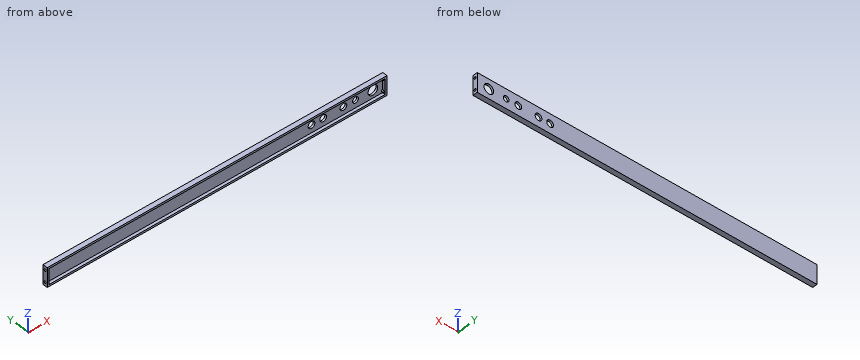
Autodesk Inventor part; units mm, degrees
ref_plane "YZ Plane" through (0, 0, 0) normal (1, 0, 0) x (0, 1, 0)
ref_plane "XZ Plane" through (0, 0, 0) normal (0, 1, 0) x (-1, 0, 0)
ref_plane "XY Plane" through (0, 0, 0) normal (0, 0, 1) x (1, 0, 0)
sketch "スケッチ1" plane through (0, 0, 0) normal (0, 0, 1) x (1, 0, 0)
  line L0 (0, 0) -> (352, 0)
  line L1 (352, 0) -> (352, 5)
  line L2 (352, 5) -> (0, 5)
  line L3 (0, 5) -> (0, 0)
  line L4 (0, 0) -> (6, 0)
  line L5 (0, 1) -> (0, 0)
  dimension "d0" = 352
  dimension "d1" = 5
extrude "押し出し1" add sketch "スケッチ1" along normal blind 20
sketch "スケッチ3" plane through (0, 0, 0) normal (-1, 0, 0) x (0, 0, 1)
  line L0 (0, 5) -> (0, 0)
  line L1 (0, 0) -> (20, 0)
  line L2 (20, 5) -> (20, 0)
  line L3 (0, 5) -> (20, 5)
  circle A0 centre (4, 2.5) radius 1.2
  circle A1 centre (16, 2.5) radius 1.2
  dimension "d14" = 2.4
  dimension "d15" = 2.4
  dimension "d16" = 2.5
  dimension "d17" = 4
  dimension "d18" = 4
  dimension "d19" = 2.5
extrude "押し出し3" cut sketch "スケッチ3" against normal blind 3 contours A0 | A1
sketch "スケッチ4" plane through (0, 0, 0) normal (0, -1, 0) x (1, 0, 0)
  line L0 (0, 0) -> (352, 0)
  line L1 (352, 0) -> (352, 20)
  line L2 (0, 20) -> (352, 20)
  line L3 (0, 0) -> (0, 20)
  line L4 (2, 2) -> (350, 2)
  line L5 (350, 2) -> (350, 18)
  line L6 (350, 18) -> (2, 18)
  line L7 (2, 18) -> (2, 2)
  dimension "d22" = 2
  dimension "d23" = 2
  dimension "d24" = 2
  dimension "d25" = 2
extrude "押し出し4" cut sketch "スケッチ4" against normal blind 3 contours L7 L6 L5 L4
sketch "スケッチ6" plane through (0, 3, 0) normal (0, -1, 0) x (1, 0, 0)
  line L0 (350, 18) -> (350, 2)
  line L1 (2, 18) -> (350, 18)
  point P0 (0, 0)
  point P1 (340, 10)
  dimension "d35" = 10
  dimension "d36" = 8
  dimension "d37" = 16
hole "穴1" at (340, 3, 10) direction (0, 1, 0) diameter 10 end through all
sketch "スケッチ7" plane through (0, 3, 0) normal (0, -1, 0) x (1, 0, 0)
  circle A0 centre (340, 10) radius 5
  line L0 (340, 10) -> (322, 10)
  point P0 (0, 0)
  dimension "d38" = 18
hole "穴2" at (322, 3, 10) direction (0, 1, 0) diameter 6 end through all
sketch "スケッチ8" plane through (0, 3, 0) normal (0, -1, 0) x (1, 0, 0)
  circle A0 centre (322, 10) radius 3
  line L0 (322, 10) -> (309.5, 10)
  point P0 (0, 0)
  dimension "d46" = 12.5
hole "穴3" at (309.5, 3, 10) direction (0, 1, 0) diameter 7 end through all
sketch "スケッチ9" plane through (0, 3, 0) normal (0, -1, 0) x (1, 0, 0)
  circle A0 centre (309.5, 10) radius 3.5
  line L0 (309.5, 10) -> (288.5, 10)
  point P0 (0, 0)
  dimension "d54" = 21
hole "穴4" at (288.5, 3, 10) direction (0, 1, 0) diameter 7 end through all
sketch "スケッチ10" plane through (0, 3, 0) normal (0, -1, 0) x (1, 0, 0)
  circle A0 centre (288.5, 10) radius 3.5
  line L0 (288.5, 10) -> (276.5, 10)
  point P0 (0, 0)
  dimension "d62" = 12
hole "穴5" at (276.5, 3, 10) direction (0, 1, 0) diameter 7 end through all
sketch "スケッチ11" plane through (352, 0, 0) normal (1, 0, 0) x (0, 0, -1)
  arc A0 (-5.0909, 3) -> (-2.9091, 3) centre (-4, 2.5) ccw
  arc A1 (-17.0909, 3) -> (-14.9091, 3) centre (-16, 2.5) ccw
  arc A2 (-14.9091, 3) -> (-17.0909, 3) centre (-16, 2.5) ccw
  arc A3 (-2.9091, 3) -> (-5.0909, 3) centre (-4, 2.5) ccw
extrude "押し出し5" cut sketch "スケッチ11" against normal blind 3
properties part number "arm1_L" material "アルミニウム 6061"
Verification items for the finished model (mm, model axes). Round coordinates to 2 decimals unless told otherwise and drop trailing zeros. Write each loop counter-clockwise with the first axis right and the second up, starting at its lowest first coordinate (ties: lowest second). Pieces come first, ordered by that corner, then holes. Notation, with made-up numbers: (52, -36) -> (86, -36) arc R30 cw to (86, 1) -> close; hole circle Ø6 at (-13, 72.5). An arc over 180 degrees is marked (long way). Write each question's results on one line, items separated by ' | '. Start each with the question number.
1. Cross-section at B-B (x = 340). Enter the section's corners in (y, z).
2. Cross-section at A-A (z = 10). Enter the section's corners in (x, y).
3. Material ranges on probe 1 along Z at (x, y) = (351.45, 2.5); probe 2 along X at (y, z) = (3.75, 10); probe 3 along X at (y, z) = (1.7, 8.5), recorded low to high. Write a range as from..to.
4. Depth check by flat-ended pin: P1, Ø6.5, axis at x = 276.5, z = 10, coming from the -Y side; P2, Ø1.5, axis at x = 217, z = 6, coming from the -Y side; P3, Ø0.8, axis at y = 3, z = 16, coming from the -X side. Enter the tip coordinate at first touch or a pass-through.
5. Cross-section at C-C (x = 51). Enter the section's corners in (y, z), then the cut area to 3 significant figures.
6. Cross-section at D-D (x = 288.5). Enter the section's corners in (y, z).
Solutions:
1) outline: (0, 0) -> (5, 0) -> (5, 5) -> (3, 5) -> (3, 2) -> (0, 2) -> close; (0, 18) -> (3, 18) -> (3, 15) -> (5, 15) -> (5, 20) -> (0, 20) -> close
2) outline: (0, 0) -> (2, 0) -> (2, 3) -> (273, 3) -> (273, 5) -> (0, 5) -> close; (280, 3) -> (285, 3) -> (285, 5) -> (280, 5) -> close; (292, 3) -> (306, 3) -> (306, 5) -> (292, 5) -> close; (313, 3) -> (319, 3) -> (319, 5) -> (313, 5) -> close; (325, 3) -> (335, 3) -> (335, 5) -> (325, 5) -> close; (345, 3) -> (350, 3) -> (350, 0) -> (352, 0) -> (352, 5) -> (345, 5) -> close
3) probe 1: z = 0..2.8, 5.2..14.8, 17.2..20 | probe 2: x = 0..273, 280..285, 292..306, 313..319, 325..335, 345..352 | probe 3: x = 0..2, 350..352
4) P1: passes through | P2: stops at y = 3 | P3: stops at x = 3
5) outline: (0, 0) -> (5, 0) -> (5, 20) -> (0, 20) -> (0, 18) -> (3, 18) -> (3, 2) -> (0, 2) -> close | area: 52.0 mm2
6) outline: (0, 0) -> (5, 0) -> (5, 6.5) -> (3, 6.5) -> (3, 2) -> (0, 2) -> close; (0, 18) -> (3, 18) -> (3, 13.5) -> (5, 13.5) -> (5, 20) -> (0, 20) -> close
